Design review of the part built by this model. Coordinates are the model's own, in mm. A direction names the side the tool comes from. Coordinates: 2 decimals unless noted, no trailing zeros. Loops run counter-clockwise (first coordinate to the right, second up) from the corner with the lowest first, then second, coordinate; pieces in that order, holes last. Notation, with made-up numbers: (86.25, 27) - (101.25, 27) arc R17 cw to (101.25, 40) - close; hole circle Ø4 at (-3, 0). An arc over 180 degrees is marked (long way). Answer in a Markdown table with one row per item. Add a question column.
(1) Clearance check with flat-ended pins moving along their axes: pin 1 (7 mm diameter, centred on y = 41.5, z = 48, fed in from +X); pin 2 (11.5 mm diameter, centred on y = 34.5, z = 64.5, fed in from -X); pin 3 (1 mm diameter, centred on x = 70.5, z = 24.5, fed in from +Y). State where each tip first meets the part, or that it passes through.
(2) For faces 1 (the face through (33.346, 41.632, -0.803)), 2 (the face through (-69.85, 39, -56)), 3 (the face through (69.85, 39, 56)), 4 (the face through (-1.536, 41.632, -146.033)), list the 3-axis set-ups (+Z, -Z, +X, -X, +Y, -Y) from which the entire face can be reached by the end or side of a thin tool; tool diameter is ignored.
(3) We need section A-A, the plane z = 41.5. Write out the cut boundary in (x, y) (3 decimals), plus the area to 3 significant figures.
(4) We need section C-C, the plane y = 19. Write out the cut boundary in (x, z) (3 decimals), plus the area to 3 significant figures.
(5) To check wall thickness, follow L1, parallel to Z at x = 39, y = 39; L2, parallel to Y at x = 96, z = 33 (3 decimals); L3, parallel to Y at x = -87, z = 119.5 (3 decimals). State the ranges of each line that lie inside material, in increasing order. Write a range as [from, to].
(6) We need section B-B, the plane x = 47. Write out the cut boundary in (y, z) (3 decimals), plus the area to 3 significant figures.
from build123d import *

# Parameters (mm, degrees)
F0_W     = 241.3
F0_H     = 311.15
F1_DEPTH = 130.175
F3_DEPTH = 311.15
F5_DEPTH = 50.8


# Not quite as in the source:
# - a length typed as a fraction of an inch, garbled in the dataset ("3 / 203.2 mm" for 3/8 in), is restored


with BuildPart() as f1:
    # F0 (on Front) → F1 (new body)
    with BuildSketch(Plane.XZ):
        Rectangle(F0_W, F0_H)
    extrude(amount=F1_DEPTH)

    # F2 (on face) → F3 (join, through all)
    with BuildSketch(Plane.XY.offset(155.575)):
        with BuildLine():
            Line((-120.65, 12.7), (-120.65, 0))
            Line((-120.65, 0), (120.65, 0))
            Line((120.65, 0), (120.65, 12.7))
            ThreePointArc((120.65, 12.7), (0, 34.925), (-120.65, 12.7))
        make_face()
    extrude(amount=-F3_DEPTH)

    # F4 (on Front) → F5 (join)
    with BuildSketch(Plane.XZ):
        with BuildLine():
            Line((69.85, 36.5125), (69.85, 76.2))
            ThreePointArc((69.85, 76.2), (0, 146.05), (-69.85, 76.2))
            Line((-69.85, 76.2), (-69.85, 36.5125))
            ThreePointArc((-69.85, 36.5125), (-33.3375, 0), (-69.85, -36.5125))
            Line((-69.85, -36.5125), (-69.85, -76.2))
            ThreePointArc((-69.85, -76.2), (0, -146.05), (69.85, -76.2))
            Line((69.85, -76.2), (69.85, -36.5125))
            ThreePointArc((69.85, -36.5125), (33.3375, 0), (69.85, 36.5125))
        make_face()
    extrude(amount=-F5_DEPTH)


solid = f1.part
Responses:
| question | item | result |
|---|---|---|
| 1 | pin 1 | stops at x = 69.85 |
| 1 | pin 2 | stops at x = -69.85 |
| 1 | pin 3 | stops at y = 27.61 |
| 2 | face 1 | +X, +Y |
| 2 | face 2 | +Z, -Z, -X, +Y |
| 2 | face 3 | +Z, -Z, +X, +Y |
| 2 | face 4 | -Z, +Y |
| 3 | outline | (-120.65, -130.175) - (120.65, -130.175) - (120.65, 12.7) arc R338.591 ccw to (69.85, 27.642) - (69.85, 50.8) - (-69.85, 50.8) - (-69.85, 27.642) arc R338.591 ccw to (-120.65, 12.7) - close |
| 3 | area | 40,600 mm2 |
| 4 | outline | (-102.618, -155.575) - (102.618, -155.575) - (102.618, 155.575) - (-102.618, 155.575) - close |
| 4 | area | 63,900 mm2 |
| 5 | L1 | z = [-134.15, -19.53], [19.53, 134.15] |
| 5 | L2 | y = [-130.175, 21.031] |
| 5 | L3 | y = [-130.175, 23.557] |
| 6 | outline | (-130.175, -155.575) - (31.647, -155.575) - (31.647, -127.872) - (50.8, -127.872) - (50.8, -28.479) - (31.647, -28.479) - (31.647, 28.479) - (50.8, 28.479) - (50.8, 127.872) - (31.647, 127.872) - (31.647, 155.575) - (-130.175, 155.575) - close |
| 6 | area | 54,200 mm2 |
